Input: part model. Units: mm. Frame: model coordinates. Coordinates: 2 decimals unless noted, no trailing zeros. Write each loop counter-clockwise with the first axis right and the second up, starting at its lowest first coordinate (ties: lowest second). Pieces come first, ordered by that corner, then holes.
1) Section query C-C (y = 1.1). Output: boundary loops of the cut face in (x, z).
2) Section query B-B (z = -4). Output: boundary loops of the cut face in (x, y).
3) Pin query (flat end, axial travel): pin 1 Ø2 at (x, z) = (3, 2.5) entering from +Y; pin 2 Ø0.5 at (x, y) = (2, 2.5) entering from +Z; pin 3 Ø0.5 at (y, z) = (2, -0.5) entering from +X. Return the tip coordinate at first contact, or that it passes through.
4) Section query D-D (z = 7). Output: boundary loops of the cut face in (x, y) (3 decimals).
5) Section query A-A (x = 0). Output: boundary loops of the cut face in (y, z).
6) Draft query along X for faces 1 (the flat face through (0, 2, 2)), 2 (the cylindrical face through (4.336, 1.282, 19.524)), 3 (the flat face through (-3, 2.6, -2)). Return one class per face: pulls with the +X half, pulls with the -X half, needs draft (parallel to the pull), parting line crosses it, or undercut.
7) Line query: L1, parallel to Y at x = -8.5, z = 3; L2, parallel to X at y = 1.9, z = -0.5; L3, parallel to Z at x = -4, y = 2.05. Output: solid intervals per line, ascending.
Autodesk Inventor part; units mm, degrees
ref_plane "YZ Plane" through (0, 0, 0) normal (1, 0, 0) x (0, 1, 0)
ref_plane "XZ Plane" through (0, 0, 0) normal (0, 1, 0) x (-1, 0, 0)
ref_plane "XY Plane" through (0, 0, 0) normal (0, 0, 1) x (1, 0, 0)
sketch "Sketch1" plane through (0, 0, 0) normal (0, 1, 0) x (-1, 0, 0)
  circle A0 centre (0, 0) radius 20
  dimension "d0" = 40
extrude "Extrusion1" add sketch "Sketch1" along normal blind 2.6
sketch "Sketch2" plane through (0, 2.6, 0) normal (0, 1, 0) x (1, 0, 0)
  line L0 (-10, -10) -> (-10, 10)
  line L1 (-10, 10) -> (10, 10)
  line L2 (10, 10) -> (10, -10)
  line L3 (10, -10) -> (-10, -10)
  line L4 (-10, -10) -> (10, 10) construction
  line L5 (-10, 10) -> (10, -10) construction
  point P0 (0, 0)
  dimension "d3" = 20
  dimension "d4" = 20
extrude "Extrusion2" cut sketch "Sketch2" against normal blind 0.6
sketch "Sketch3" plane through (0, 2, 0) normal (0, 1, 0) x (1, 0, 0)
  line L0 (-5.9162, 8.3364) -> (5.9889, 8.3364) construction
  line L1 (5.9889, 8.3364) -> (5.9889, -8.2636) construction
  line L2 (5.9889, -8.2636) -> (-5.9162, -8.2636) construction
  line L3 (-5.9162, -8.2636) -> (-5.9162, 8.3364) construction
  line L4 (5.693, 6.3723) -> (-2.0286, 6.3723)
  line L5 (-2.0286, 6.3723) -> (-2.0286, 1.691)
  line L6 (-2.0286, 1.691) -> (5.3701, 1.691)
  line L7 (5.3701, 1.691) -> (5.3701, -0.273)
  line L8 (5.3701, -0.273) -> (-2.0286, -0.273)
  line L9 (-2.0286, -0.273) -> (-2.0286, -8.2636)
  line L10 (-2.0286, -8.2636) -> (-4.2347, -8.2636)
  line L11 (-4.2347, -8.2636) -> (-4.2347, 8.3364)
  line L12 (-4.2347, 8.3364) -> (5.693, 8.3364)
  line L13 (5.693, 8.3364) -> (5.693, 6.3723)
  point P0 (0, 0)
extrude "Extrusion3" add sketch "Sketch3" along normal blind 0.6
properties part number "TopMarkerPreset"
Answer:
1. outline: circle Ø40 at (0, 0)
2. outline: (-19.6, 0) - (19.6, 0) - (19.6, 2.6) - (10, 2.6) - (10, 2) - (-2.03, 2) - (-2.03, 2.6) - (-4.23, 2.6) - (-4.23, 2) - (-10, 2) - (-10, 2.6) - (-19.6, 2.6) - close
3. pin 1: stops at y = 2
3. pin 2: stops at z = 19.92
3. pin 3: stops at x = 20
4. outline: (-18.735, 0) - (18.735, 0) - (18.735, 2.6) - (10, 2.6) - (10, 2) - (-2.029, 2) - (-2.029, 2.6) - (-4.235, 2.6) - (-4.235, 2) - (-10, 2) - (-10, 2.6) - (-18.735, 2.6) - close
5. outline: (0, -20) - (2.6, -20) - (2.6, -10) - (2, -10) - (2, -8.34) - (2.6, -8.34) - (2.6, -6.37) - (2, -6.37) - (2, -1.69) - (2.6, -1.69) - (2.6, 0.27) - (2, 0.27) - (2, 10) - (2.6, 10) - (2.6, 20) - (0, 20) - close
6. face 1: undercut
6. face 2: parting line crosses it
6. face 3: needs draft
7. L1: y = 0 to 2
7. L2: x = -19.99 to 19.99
7. L3: z = -19.6 to -10, -8.34 to 8.26, 10 to 19.6
